For this review, take the finished solid that the model builds, in its own axes (mm). A direction names the side the tool comes from. Round coordinates to 2 decimals unless told otherwise and drop trailing zeros. Order: outer loops, then holes, each group sorted by start corner. A loop starts at its lowest first (then second) coordinate and runs counter-clockwise, first axis right, second up. Notation, with made-up numbers: (-33, 73.5) - (13, 73.5) arc R16 cw to (13, 103.5) - close; hole circle Ø7 at (35, 38.25). An arc over 180 degrees is marked (long way). One line per question, with ' | ' between items.
```python
from build123d import *

# Parameters (mm, degrees)
SKETCH_1_R               = 60
EXTRUDE_1_DEPTH          = 28
SKETCH_2_R               = 48.25
CUT_EXTRUDE_1_DEPTH      = 90.353231615
SKETCH_4_R               = 150
EXTRUDE_3_DEPTH          = 10
SKETCH_5_R               = 35
CUT_EXTRUDE_2_DEPTH      = 216.50870052
SKETCH_6_R               = 2
CUT_EXTRUDE_3_DEPTH      = 216.50870052
PATTERN_CIRCULAR_1_COUNT = 6
EXTRUDE_START            = 15
SKETCH_7_R               = 170
SKETCH_7_R_2             = 48.25
EXTRUDE_4_DEPTH          = 15
SKETCH_9_R               = 2
CUT_EXTRUDE_4_DEPTH      = 244.40090386
PATTERN_CIRCULAR_2_COUNT = 8
CUT_EXTRUDE_5_DEPTH      = 10


with BuildPart() as part:
    # 草图1 → 凸台-拉伸1 (new body)
    with BuildSketch(Plane.XY):
        Circle(SKETCH_1_R)
    extrude(amount=EXTRUDE_1_DEPTH)

    # 草图2 → 切除-拉伸1 (cut, through all)
    with BuildSketch(Plane.XY.offset(28)):
        Circle(SKETCH_2_R)
    extrude(amount=-CUT_EXTRUDE_1_DEPTH, mode=Mode.SUBTRACT)

    # 草图4 → 凸台-拉伸3 (add)
    with BuildSketch(Plane.XY.offset(28)):
        Circle(SKETCH_4_R)
    extrude(amount=EXTRUDE_3_DEPTH)

    # 草图5 → 切除-拉伸2 (cut, through all)
    with BuildSketch(Plane.XY.offset(38)):
        Circle(SKETCH_5_R)
    extrude(amount=-CUT_EXTRUDE_2_DEPTH, mode=Mode.SUBTRACT)

    # 草图6 → 切除-拉伸3 (cut, through all)
    with BuildSketch(Plane.XY.offset(38)):
        with Locations((0, 42.356738024)):
            Circle(SKETCH_6_R)
    cut_extrude_3 = extrude(amount=-CUT_EXTRUDE_3_DEPTH, mode=Mode.SUBTRACT)

    # 阵列(圆周)1: 切除-拉伸3 ×6 about axis
    pattern_circular_1_axis = Axis((0, 0, 0), (0, 0, 1))
    for i in range(1, PATTERN_CIRCULAR_1_COUNT):
        add(cut_extrude_3.rotate(pattern_circular_1_axis, i * 360 / PATTERN_CIRCULAR_1_COUNT), mode=Mode.SUBTRACT)

    # 草图7 → 凸台-拉伸4 (add)
    with BuildSketch(Plane.XY.offset(38).offset(EXTRUDE_START)):
        Circle(SKETCH_7_R)
        Circle(SKETCH_7_R_2, mode=Mode.SUBTRACT)
    extrude(amount=-EXTRUDE_4_DEPTH)

    # 草图9 → 切除-拉伸4 (cut, through all)
    with BuildSketch(Plane(origin=(0, 0, 38), x_dir=(-1, 0, 0), z_dir=(0, 0, -1))):
        with Locations((0, 160)):
            Circle(SKETCH_9_R)
    cut_extrude_4 = extrude(amount=-CUT_EXTRUDE_4_DEPTH, mode=Mode.SUBTRACT)

    # 阵列(圆周)2: 切除-拉伸4 ×8 about axis
    pattern_circular_2_axis = Axis((0, 0, 0), (0, 0, 1))
    for i in range(1, PATTERN_CIRCULAR_2_COUNT):
        add(cut_extrude_4.rotate(pattern_circular_2_axis, i * 360 / PATTERN_CIRCULAR_2_COUNT), mode=Mode.SUBTRACT)

    # 草图11 → 切除-拉伸5 (cut)
    with BuildSketch(Plane.XY.offset(53)):
        with BuildLine():
            Line((47.645322741, -7.614835578), (167.869530902, -26.829472503))
            ThreePointArc((167.869530902, -26.829472503), (165.346802936, -39.502338652), (161.868807028, -51.946985586))
            Line((161.868807028, -51.946985586), (45.810704842, -15.147337122))
            ThreePointArc((45.810704842, -15.147337122), (46.879546902, -11.417993791), (47.645322741, -7.614835578))
        make_face()
        with BuildLine():
            Line((-45.810704842, 15.147337122), (-161.405592189, 53.368856183))
            ThreePointArc((-161.405592189, 53.368856183), (-165.171460589, 40.229200923), (-167.869530902, 26.829472503))
            Line((-167.869530902, 26.829472503), (-47.645322741, 7.614835578))
            ThreePointArc((-47.645322741, 7.614835578), (-46.879546902, 11.417993791), (-45.810704842, 15.147337122))
        make_face()
    extrude(amount=-CUT_EXTRUDE_5_DEPTH, mode=Mode.SUBTRACT)


solid = part.part
```
(1) Mouldability with a two-part tool opening along X and no side actions: class faces 4 (the cylindrical face through (-19.527, 148.724, 32.93)), 5 (the flat face through (121, -29, 43)), 6 (the flat face through (-40.3, 26.9, 0)) as released by +X, released by -X, zero draft, split by the parting line, or undercut.
Output values:
face 4: split by the parting line | face 5: undercut | face 6: zero draft
(2) We need section D-D on x = -137.5. State the section outline as (y, z) points, plus the area to 3 significant figures.
Output values:
outline: (-99.97, 38) - (-59.95, 38) - (-59.95, 28) - (59.95, 28) - (59.95, 38) - (99.97, 38) - (99.97, 53) - (45.46, 53) - (45.46, 43) - (21.98, 43) - (21.98, 53) - (-99.97, 53) - close | area: 3,960 mm^2
(3) We need section A-A on x = 28. State the section outline as (y, z) points, plus the area to 3 significant figures.
Output values:
outline: (-167.68, 38) - (-147.36, 38) - (-147.36, 28) - (-53.07, 28) - (-53.07, 0) - (-39.29, 0) - (-39.29, 28) - (-21, 28) - (-21, 38) - (-39.29, 38) - (-39.29, 53) - (-167.68, 53) - close; (21, 28) - (39.29, 28) - (39.29, 0) - (53.07, 0) - (53.07, 28) - (147.36, 28) - (147.36, 38) - (167.68, 38) - (167.68, 53) - (39.29, 53) - (39.29, 38) - (21, 38) - close | area: 7,150 mm^2
(4) We need section B-B on z = 32. State the section outline as (x, y) points, plus the area to 3 significant figures.
Output values:
outline: circle Ø300 at (0, 0); hole circle Ø4 at (-36.68, -21.18); hole circle Ø4 at (-36.68, 21.18); hole circle Ø70 at (0, 0); hole circle Ø4 at (0, -42.36); hole circle Ø4 at (0, 42.36); hole circle Ø4 at (36.68, -21.18); hole circle Ø4 at (36.68, 21.18) | area: 66,800 mm^2
(5) Insertion check: pin 1 (5 mm diameter, centred on x = 36.5, z = 43.5, fed in from +Y); pin 2 (10 mm diameter, centred on y = 27.5, z = 29.5, fed in from +X); pin 3 (6.5 mm diameter, centred on x = 0, y = -160, fed in from -Z). Each pin has a flat end and moves straight along its axis. Give the tip position at first contact, or say it passes through.
Output values:
pin 1: y = 166.57 | pin 2: x = 148.3 | pin 3: z = 38
(6) For faces 1 (the flat face through (-121, 31, 43)), 2 (the flat face through (-0.8, -150.3, 38)), 3 (the flat face through (2, 73, 53)), list the 3-axis set-ups (+Z, -Z, +X, -X, +Y, -Y) from which the entire face can be reached by the end or side of a thin tool; tool diameter is ignored.
Output values:
face 1: +Z | face 2: -Z | face 3: +Z, +X, -X, +Y, -Y
(7) For probe 1 along X at (y, z) = (0, 43); probe 2 along Z at (x, y) = (-16.5, -120); probe 3 along X at (y, z) = (28.5, 4), list the stretches that pass through material, from the lowest coordinate up. Write a range as [from, to].
Output values:
probe 1: [-170, -162], [-158, -48.25], [48.25, 158], [162, 170] | probe 2: [28, 53] | probe 3: [-52.8, -38.93], [38.93, 52.8]
(8) We need section C-C on y = 88.5. State the section outline as (x, z) points, plus the area to 3 significant figures.
Output values:
outline: (-145.15, 38) - (-121.11, 38) - (-121.11, 28) - (121.11, 28) - (121.11, 38) - (145.15, 38) - (145.15, 53) - (-145.15, 53) - close | area: 6,780 mm^2
